The model under review builds one solid part; all positions refer to its coordinate system, in mm. A direction names the side the tool comes from. Coordinates: 2 decimals unless noted, no trailing zeros. Write each loop counter-clockwise with the first axis right and the second up, starting at its lowest first coordinate (ties: lowest second). Pieces come first, ordered by that corner, then holes. Notation, with made-up numbers: (10.5, -27) - (29.5, -27) arc R33 ccw to (29.5, 10) - close; hole circle Ø10 at (-19, 65.5). An arc over 180 degrees is marked (long way). Put each result on its own line as item: value. Start each with the question number.
Item 1: Consider section B-B on x = 0. Give the boundary of the cut face in (y, z), then the cut area to 3 significant figures.
Item 2: Mouldability with a two-part tool opening along Z and no side actions: class faces 3 (the face through (-4.146, -3.157, -2.157)), 4 (the face through (-7.75, 12.91, -1.72)), 5 (the face through (-3.1, 0.127, 1.1)), 6 (the face through (2.3, -6.35, -4.3)) as pulls with the +Z half, pulls with the -Z half, needs draft (parallel to the pull), parting line crosses it, or undercut.
Item 3: Consider section C-C on y = -0.5. Give the boundary of the cut face in (x, z) (1 decimal).
Item 4: To check wall thickness, follow L1, parallel to X at y = -1.75, z = 0; L2, parallel to X at y = 13, z = 0; L3, parallel to Y at x = 5.5, z = 6.75. State the ranges of each line that lie inside material, in increasing order. Write a range as [from, to].
Item 5: Consider section D-D on y = 7.5. Give the boundary of the cut face in (x, z) (1 decimal).
Item 6: For pin 1 (12 mm diameter, centred on x = -10.5, y = -1, fed in from -Z); pin 2 (8 mm diameter, centred on y = 11, z = -3, fed in from +X); pin 3 (2 mm diameter, centred on y = 8, z = 6, fed in from -X), all flat-tipped, find the tip position at first contact; note any pin that passes through.
Item 7: Consider section A-A on z = 0. Give the boundary of the cut face in (x, y), then the cut area to 3 significant figures.
Item 8: Machinability: for faces 1 (the face through (-6, 0, -6)), 2 (the face through (0.628, -2.348, 14.274)), which of the approach directions +Z, -Z, +X, -X, +Y, -Y give a long, thin tool a straight path to every point of the face, cutting with its end or side? Answer none if there is none.
```python
from build123d import *

# Parameters (mm, degrees)
SKETCH1_R           = 7.9375
SKETCH1_R_2         = 3.1115
BOSS_EXTRUDE1_DEPTH = 26.19375
SKETCH2_R           = 14.2875
BOSS_EXTRUDE2_DEPTH = 6.35
CHAMFER1_SIZE       = 1.5875
CHAMFER1_SIZE2      = 4.361620403
SKETCH3_R           = 4.6736
CUT_EXTRUDE1_DEPTH  = 6.477


with BuildPart() as part:
    # Sketch1 → Boss-Extrude1 (new body)
    with BuildSketch(Plane(origin=(0, 0, 0), x_dir=(1, 0, 0), z_dir=(0, 1, 0))):
        with Locations(Location((0, 0, 0), (0, 0, 270))):
            Circle(SKETCH1_R)
        with Locations(Location((0, 0, 0), (0, 0, 270))):
            Circle(SKETCH1_R_2, mode=Mode.SUBTRACT)
    extrude(amount=BOSS_EXTRUDE1_DEPTH)

    # Sketch2 → Boss-Extrude2 (add)
    with BuildSketch(Plane.XZ):
        with Locations(Location((0, 0, 0), (0, 0, 270))):
            Circle(SKETCH2_R)
    extrude(amount=BOSS_EXTRUDE2_DEPTH)

    # Chamfer1
    chamfer1_edges = [part.edges().sort_by_distance(p)[0] for p in [
        (0, -6.35, 14.2875),
    ]]
    chamfer1_side = [part.faces().sort_by_distance(p)[0] for p in [
        (0, -3.175, 14.2875),
    ]]
    chamfer(chamfer1_edges, length=CHAMFER1_SIZE, length2=CHAMFER1_SIZE2, reference=chamfer1_side[0])

    # Sketch3 → Cut-Extrude1 (cut)
    with BuildSketch(Plane.XZ.offset(6.35)):
        with Locations(Location((0, 0, 0), (0, 0, 270))):
            Circle(SKETCH3_R)
    extrude(amount=-CUT_EXTRUDE1_DEPTH, mode=Mode.SUBTRACT)


solid = part.part
```
Report:
1. outline: (-6.35, -9.93) - (-4.76, -14.29) - (0, -14.29) - (0, -7.94) - (26.19, -7.94) - (26.19, -3.11) - (0.13, -3.11) - (0.13, -4.67) - (-6.35, -4.67) - close; (-6.35, 4.67) - (0.13, 4.67) - (0.13, 3.11) - (26.19, 3.11) - (26.19, 7.94) - (0, 7.94) - (0, 14.29) - (-4.76, 14.29) - (-6.35, 9.93) - close
1. area: 368 mm²
2. face 3: undercut
2. face 4: parting line crosses it
2. face 5: undercut
2. face 6: needs draft
3. outline: circle Ø28.6 at (0, 0); hole circle Ø9.3 at (0, 0)
4. L1: [-14.29, -4.67], [4.67, 14.29]
4. L2: [-7.94, -3.11], [3.11, 7.94]
4. L3: [-6.35, 0]
5. outline: circle Ø15.9 at (0, 0); hole circle Ø6.2 at (0, 0)
6. pin 1: z = -13.56
6. pin 2: x = 7.94
6. pin 3: x = -6.16
7. outline: (-14.29, -4.76) - (-9.93, -6.35) - (-4.67, -6.35) - (-4.67, 0.13) - (-3.11, 0.13) - (-3.11, 26.19) - (-7.94, 26.19) - (-7.94, 0) - (-14.29, 0) - close; (3.11, 0.13) - (4.67, 0.13) - (4.67, -6.35) - (9.93, -6.35) - (14.29, -4.76) - (14.29, 0) - (7.94, 0) - (7.94, 26.19) - (3.11, 26.19) - close
7. area: 368 mm²
8. face 1: +Y
8. face 2: +Y, -Y
